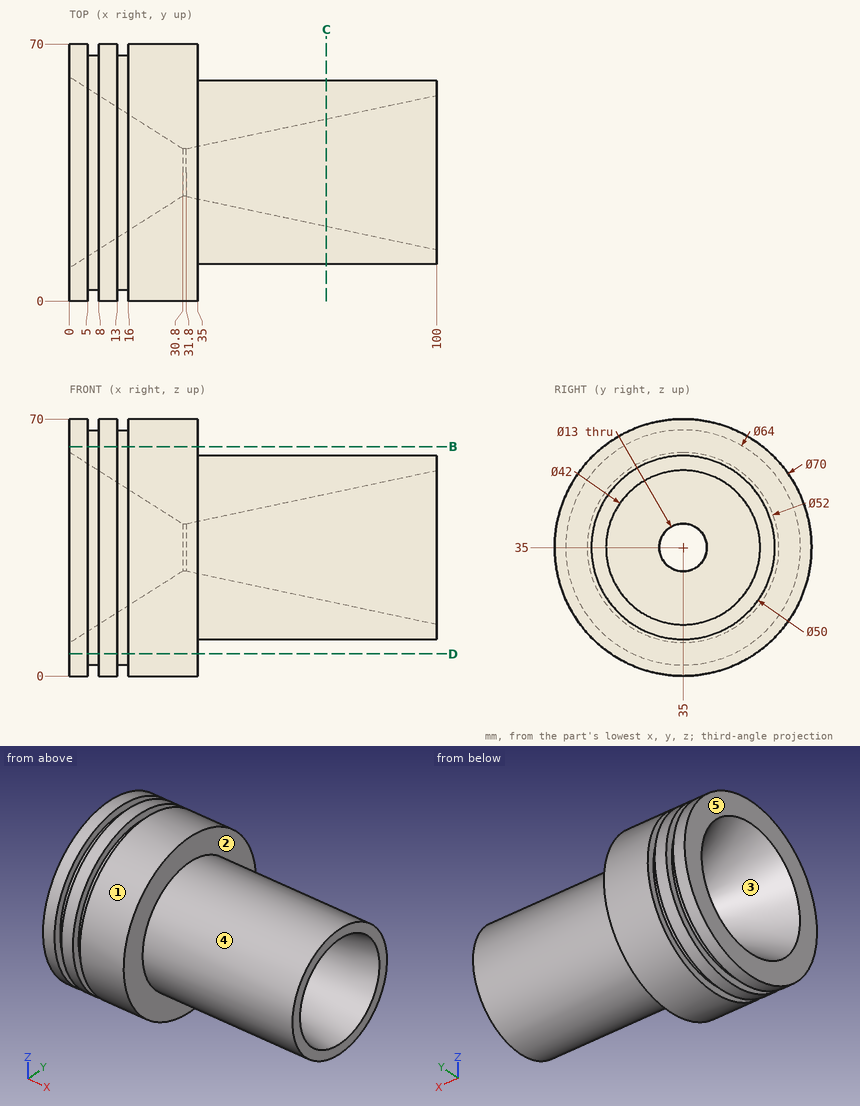
Design review of the part shown in the three views and the two pictorial views. Dimensions are in mm from the part's minimum x, y and z. A direction names the side the tool comes from. Round coordinates to 2 decimals unless told otherwise and drop trailing zeros. Order: outer loops, then holes, each group sorted by start corner. A loop starts at its lowest first (then second) coordinate and runs counter-clockwise, first axis right, second up.
Q1. We need section B-B, the plane z = 62.5. Give the boundary of the cut face in (x, y).
Findings below:
outline: (0, 13.35) - (5, 13.35) - (5, 18.64) - (8, 18.64) - (8, 13.35) - (13, 13.35) - (13, 18.64) - (16, 18.64) - (16, 13.35) - (35, 13.35) - (35, 56.65) - (16, 56.65) - (16, 51.36) - (13, 51.36) - (13, 56.65) - (8, 56.65) - (8, 51.36) - (5, 51.36) - (5, 56.65) - (0, 56.65) - close
Q2. Wall thickness on line 1 (Z direction, x = 31.2, y = 35); line 2 (X direction, y = 66, z = 45): over which ranges is each line inside the solid? List them lowest first.
Findings below:
line 1: z = 0 to 28.5, 41.5 to 70
line 2: x = 0 to 5, 8 to 13, 16 to 35
Q3. Mouldability with a two-part tool opening along Y and no side actions: class the marked faces 3, 4 and 5 as pulls with the +Y half, pulls with the -Y half, needs draft (parallel to the pull), parting line crosses it, or undercut.
Findings below:
face 3: undercut
face 4: parting line crosses it
face 5: needs draft
Q4. We need section D-D, the plane z = 6. Give the boundary of the cut face in (x, y).
Findings below:
outline: (0, 15.4) - (5, 15.4) - (5, 21.47) - (8, 21.47) - (8, 15.4) - (13, 15.4) - (13, 21.47) - (16, 21.47) - (16, 15.4) - (35, 15.4) - (35, 54.6) - (16, 54.6) - (16, 48.53) - (13, 48.53) - (13, 54.6) - (8, 54.6) - (8, 48.53) - (5, 48.53) - (5, 54.6) - (0, 54.6) - close
Q5. Insertion check: P1, Ø4, axis at y = 53.5, z = 10, coming from the +X side; P2, Ø1.5, axis at x = 47, z = 37.5, coming from the +Y side; P3, Ø6, axis at x = 39, z = 28.5, coming from the -Y side. Each pin has a flat end and moves straight along its axis. Give the tip position at first contact, or say it passes through.
Findings below:
P1: stops at x = 35
P2: stops at y = 59.94
P3: stops at y = 10.25
Q6. We need section C-C, the plane x = 70. Give the boundary of the cut face in (y, z).
Findings below:
outline: circle Ø50 at (35, 35); hole circle Ø29.24 at (35, 35)
Q7. Machinability: for the marked faces 1 and 2, which of the approach directions +Z, -Z, +X, -X, +Y, -Y give a long, thin tool a straight path to every point of the face, cutting with its end or side? Answer none if there is none.
Findings below:
face 1: +X, -X
face 2: +X
